from build123d import *

# Parameters (mm, degrees)
CROQUIS1_W              = 33.25
CROQUIS1_H              = 197
SALIENTE_EXTRUIR1_DEPTH = 5
CROQUIS2_R              = 1.5
CORTAR_EXTRUIR1_DEPTH   = 15
CROQUIS3_W              = 25
CROQUIS3_H              = 2.5
SALIENTE_EXTRUIR2_DEPTH = 4
REDONDEO2_R             = 1


with BuildPart() as part:
    # Croquis1 → Saliente-Extruir1 (new body)
    with BuildSketch(Plane.XY):
        Rectangle(CROQUIS1_W, CROQUIS1_H)
    extrude(amount=SALIENTE_EXTRUIR1_DEPTH)

    # Croquis2 → Cortar-Extruir1 (cut)
    with BuildSketch(Plane(origin=(0, 98.5, 0), x_dir=(1, 0, 0), z_dir=(0, 1, 0))):
        with Locations(Location((0, -2.5, 0), (0, 0, 180))):
            Circle(CROQUIS2_R)
    extrude(amount=-CORTAR_EXTRUIR1_DEPTH, mode=Mode.SUBTRACT)

    # Croquis3 → Saliente-Extruir2 (add)
    with BuildSketch(Plane.XZ.offset(98.5)):
        with Locations((0, 2.5)):
            Rectangle(CROQUIS3_W, CROQUIS3_H)
    extrude(amount=SALIENTE_EXTRUIR2_DEPTH)

    # Redondeo2
    redondeo2_edges = [part.edges().sort_by_distance(p)[0] for p in [
        (-12.5, -100.5, 3.75),
        (-12.5, -100.5, 1.25),
        (12.5, -100.5, 1.25),
        (12.5, -100.5, 3.75),
    ]]
    fillet(redondeo2_edges, radius=REDONDEO2_R)


solid = part.part
Source: CAD feature listing. Evaluate the final solid. Frame: model axes, mm. A direction names the side the tool comes from. Coordinates: 2 decimals unless noted, no trailing zeros. Answer in a Markdown table with one row per item.
Q1. First-contact query: pin 1 (4.5 mm diameter, centred on x = 0.5, y = -101, fed in from +Z); pin 2 (0.9 mm diameter, centred on x = -0.5, z = 2.5, fed in from +Y); pin 3 (2 mm diameter, centred on x = 4.5, y = -100, fed in from -Z). Flat tips, straight axial feed; report the tip coordinate or a pass-through.
Answers below:
| item | result |
|---|---|
| pin 1 | stops at z = 3.75 |
| pin 2 | stops at y = 83.5 |
| pin 3 | stops at z = 1.25 |
Q2. Ray query, probe 1 along Z at (x, y) = (0, 91.75); probe 2 along Y at (x, z) = (-14.5, 2.55); probe 3 along Y at (x, z) = (1, 2.9). Return the intervals inside material, ascending. Write a range as from..to.
Answers below:
| item | result |
|---|---|
| probe 1 | z = 0..1, 4..5 |
| probe 2 | y = -98.5..98.5 |
| probe 3 | y = -102.5..83.5 |
Q3. Set-up query: faces 1 (the flat face through (16.625, -1, 2)), 2 (the flat face through (0, -100, 1.25)), 3 (the flat face through (0, -100, 3.75)). Return all of +Z, -Z, +X, -X, +Y, -Y with unobstructed straight access to the full face (end or side cutting, diameter ignored); none if empty.
Answers below:
| item | result |
|---|---|
| face 1 | +Z, -Z, +X, +Y, -Y |
| face 2 | -Z, +X, -X, -Y |
| face 3 | +Z, +X, -X, -Y |
